Print and shaded views of the part. All mm, measured from the part's lowest x, y and z. A direction names the side the tool comes from. Round coordinates to 2 decimals unless told otherwise and drop trailing zeros. Loops run counter-clockwise (first coordinate to the right, second up) from the corner with the lowest first, then second, coordinate; pieces in that order, holes last. Notation, with made-up numbers: (-14.5, 46) - (23.5, 46) arc R18 ccw to (23.5, 61) - close; hole circle Ø10 at (-0.75, 14.25). An arc over 180 degrees is marked (long way). Answer as a JSON object with one key per item and string values.
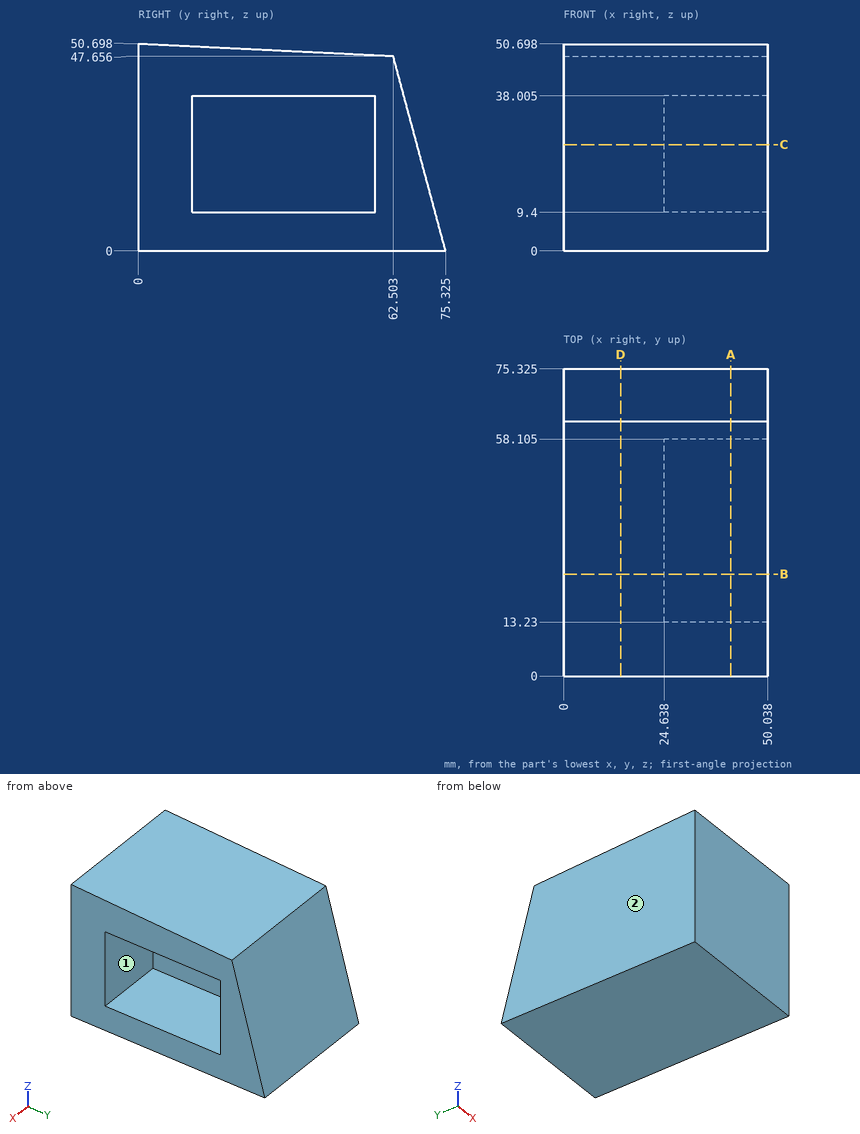
1) Drop flat-ended pins along their axis: P1, Ø2, axis at x = 18.5, z = 35.5, coming from the +Y side; P2, Ø3, axis at y = 27, z = 27.5, coming from the -X side; P3, Ø8.5, axis at y = 30, z = 24.5, coming from the +X side; P4, Ø12.5, axis at x = 39.5, z = 18, coming from the +Y side. Give the stop position or say it passes through.
Values follow:
{"P1": "y = 66.04", "P2": "x = 0", "P3": "x = 24.64", "P4": "y = 72.16"}
2) Slice it at B-B on y = 25. List the corners of the cut face in (x, z) (1 decimal).
Values follow:
{"outline": "(0, 0) - (50, 0) - (50, 9.4) - (24.6, 9.4) - (24.6, 38) - (50, 38) - (50, 49.5) - (0, 49.5) - close"}
3) Slice it at C-C on z = 26. List the corners of the cut face in (x, y) (1 decimal).
Values follow:
{"outline": "(0, 0) - (50, 0) - (50, 13.2) - (24.6, 13.2) - (24.6, 58.1) - (50, 58.1) - (50, 68.3) - (0, 68.3) - close"}
4) Slice it at A-A on x = 41. List the corners of the cut face in (y, z) (1 decimal).
Values follow:
{"outline": "(0, 0) - (75.3, 0) - (62.5, 47.7) - (0, 50.7) - close; hole (13.2, 9.4) - (58.1, 9.4) - (58.1, 38) - (13.2, 38) - close"}
5) Tool access for the marked faces 1 and 2: list every direction of +Z, -Z, +X, -X, +Y, -Y with a clear straight run to the whole face (end or side of a thin tool).
Values follow:
{"face 1": "+X", "face 2": "+Z, -Z, -X, +Y, -Y"}
6) Slice it at D-D on x = 14. List the corners of the cut face in (y, z) (1 decimal).
Values follow:
{"outline": "(0, 0) - (75.3, 0) - (62.5, 47.7) - (0, 50.7) - close"}
7) Probe probe 1 along Y at (x, z) = (47, 25) (1 decimal); probe 2 along Z at (x, y) = (29.5, 17) (1 decimal); probe 3 along Y at (x, z) = (43, 9.5) (1 decimal). List the from-to ranges inside material, lowest first.
Values follow:
{"probe 1": "0 to 13.2, 58.1 to 68.6", "probe 2": "0 to 9.4, 38 to 49.9", "probe 3": "0 to 13.2, 58.1 to 72.8"}
